from build123d import *

# Parameters (mm, degrees)
SKETCH_2_R          = 7.75
CUT_EXTRUDE_1_DEPTH = 1.75
SKETCH_3_R          = 3.9
EXTRUDE_1_DEPTH     = 2.5
CUT_EXTRUDE_2_REACH = 18.21
SKETCH_4_R          = 2


with BuildPart() as part:
    # 草图1 → 旋转1 (revolve)
    with BuildSketch(Plane.XY):
        Polygon((0, 0), (-8, 0), (-8, 0.5), (-8.5, 0.5), (-8.5, 1), (-10.5, 2), (-10.5, 2.5), (0, 2.5), align=None)
    revolve_1 = revolve(axis=Axis((0, 2.5, 0), (0, -1, 0)))

    # 镜向1: 旋转1 across plane
    add(revolve_1.mirror(Plane.ZX))

    # 草图2 → 切除-拉伸1 (cut)
    with BuildSketch(Plane(origin=(0, 2.5, 0), x_dir=(1, 0, 0), z_dir=(0, 1, 0))):
        with Locations(Location((0, 0, 0), (0, 0, 180))):
            Circle(SKETCH_2_R)
    cut_extrude_1 = extrude(amount=-CUT_EXTRUDE_1_DEPTH, mode=Mode.SUBTRACT)

    # 草图3 → 凸台-拉伸1 (add)
    with BuildSketch(Plane(origin=(0, 0.75, 0), x_dir=(1, 0, 0), z_dir=(0, 1, 0))):
        with Locations(Location((0, 0, 0), (0, 0, 180))):
            Circle(SKETCH_3_R)
    extrude_1 = extrude(amount=EXTRUDE_1_DEPTH)

    # 镜向2: 切除-拉伸1, 凸台-拉伸1 across plane
    add(cut_extrude_1.mirror(Plane.ZX), mode=Mode.SUBTRACT)
    add(extrude_1.mirror(Plane.ZX))

    # 草图4 → 切除-拉伸2 (cut, up to next)
    with BuildSketch(Plane(origin=(0, 3.25, 0), x_dir=(1, 0, 0), z_dir=(0, 1, 0)), mode=Mode.PRIVATE) as cut_extrude_2_sk1:
        with Locations(Location((0, 0, 0), (0, 0, 180))):
            Circle(SKETCH_4_R)
    cut_extrude_2_tool1 = extrude(cut_extrude_2_sk1.sketch, amount=-CUT_EXTRUDE_2_REACH, mode=Mode.PRIVATE) & part.part
    add(cut_extrude_2_tool1.solids().sort_by_distance((0, 3.25, 0))[0], mode=Mode.SUBTRACT)


solid = part.part
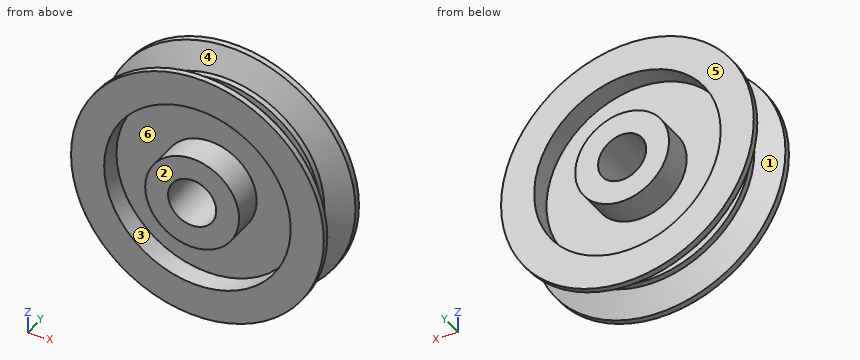
Could you check a few things on this model? Use its own coordinates, in mm. Face numbers are marked on the shaded views. A direction names the side the tool comes from. Round coordinates to 2 decimals unless told otherwise and drop trailing zeros. Order: outer loops, then holes, each group sorted by start corner. A loop starts at its lowest first (then second) coordinate and runs counter-clockwise, first axis right, second up.
(1) Which directions (+Z, -Z, +X, -X, +Y, -Y) give clear straight access to the entire face, cutting with the end or side of a thin tool? Please do the marked faces 4, 5 and 6.
Response values:
face 4: none
face 5: +Y
face 6: -Y
(2) Imagine slicing it at B-B (y = 2.75). Write out the boundary of the cut face in (x, z), plus the area to 3 significant figures.
Response values:
outline: circle Ø7.8 at (0, 0); hole circle Ø4 at (0, 0)
area: 35.2 mm2
(3) If we mould it in two halves opening along Y, with no side actions, what happens to the marked faces 1, 2 and 3? For each: released by +Y, released by -Y, zero draft, split by the parting line, or undercut.
Response values:
face 1: undercut
face 2: released by -Y
face 3: zero draft
(4) Please list where these lines run through material, in increasing order: line 1 along Z through (x, y) = (0, 2.1); line 2 along Z through (x, y) = (0, 1.8); line 3 along Y through (x, z) = (1, 7.25).
Response values:
line 1: z = -10.5 to -7.75, -3.9 to -2, 2 to 3.9, 7.75 to 10.5
line 2: z = -10.1 to -7.75, -3.9 to -2, 2 to 3.9, 7.75 to 10.1
line 3: y = -0.75 to 0.75
(5) I'm going to push flat-ended pins straight in: pin 1 (3 mm diameter, centred on y = -2, z = -6, fed in from +X); pin 2 (2.5 mm diameter, centred on x = 0, z = 0, fed in from +Y); pin 3 (1 mm diameter, centred on x = -1.5, z = -5, fed in from +Y); pin 4 (3 mm diameter, centred on x = -4.5, z = 8, fed in from -Y). Where does each tip first touch, or does it pass through?
Response values:
pin 1: stops at x = 9.49
pin 2: passes through
pin 3: stops at y = 0.75
pin 4: stops at y = -2.5
(6) Imagine slicing it at A-A (y = -1.75). Write out the boundary of the cut face in (x, z), plus the area to 3 significant figures.
Response values:
outline: circle Ø20 at (0, 0); circle Ø7.8 at (0, 0); hole circle Ø15.5 at (0, 0); hole circle Ø4 at (0, 0)
area: 161 mm2
